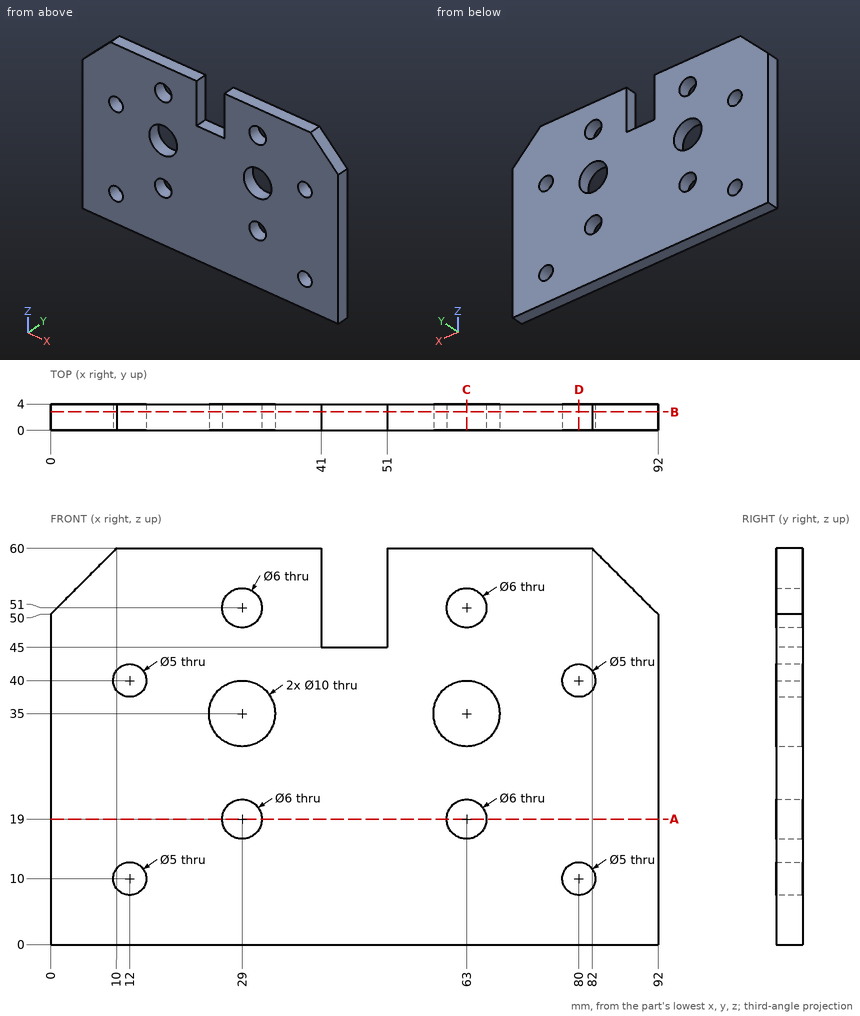
Check sheet for the drawn part. Datum: minimum x, y, z corner. Units: mm. Round coordinates to 2 decimals unless told otherwise and drop trailing zeros. Loops run counter-clockwise (first coordinate to the right, second up) from the corner with the lowest first, then second, coordinate; pieces in that order, holes last.
Item 1: Gauge pin test, flat ends, axial feed: pin 1 (7 mm diameter, centred on x = 63, z = 19, fed in from -Y); pin 2 (5.5 mm diameter, centred on x = 63, z = 51, fed in from -Y) (1 decimal); pin 3 (2 mm diameter, centred on y = 2, z = 53, fed in from -X); pin 4 (1.2 mm diameter, centred on y = 2.5, z = 54, fed in from +X). Record the tip position at first contact, or that the pin passes through.
Item 2: Cross-section at C-C on x = 63. Record the boundary of the cut face in (y, z), then the cut area to 3 significant figures.
Item 3: Cross-section at D-D on x = 80. Record the boundary of the cut face in (y, z).
Item 4: Thickness scan on line 1 (X direction, y = 1.2, z = 35); line 2 (X direction, y = 1.2, z = 19); line 3 (X direction, y = 0.6, z = 47). Record the ranges inside material, lowest first.
Item 5: Cross-section at A-A on z = 19. Record the boundary of the cut face in (x, y).
Item 6: Cross-section at B-B on y = 2.8. Count the separate pieces of the cut face and the enclosed holes in it, then the cut area to 3 significant figures.
Answer sheet:
1. pin 1: stops at y = 0
1. pin 2: passes through
1. pin 3: stops at x = 2
1. pin 4: stops at x = 88.6
2. outline: (0, 0) - (4, 0) - (4, 16) - (0, 16) - close; (0, 22) - (4, 22) - (4, 30) - (0, 30) - close; (0, 40) - (4, 40) - (4, 48) - (0, 48) - close; (0, 54) - (4, 54) - (4, 60) - (0, 60) - close
2. area: 152 mm2
3. outline: (0, 0) - (4, 0) - (4, 7.5) - (0, 7.5) - close; (0, 12.5) - (4, 12.5) - (4, 37.5) - (0, 37.5) - close; (0, 42.5) - (4, 42.5) - (4, 60) - (0, 60) - close
4. line 1: x = 0 to 24, 34 to 58, 68 to 92
4. line 2: x = 0 to 26, 32 to 60, 66 to 92
4. line 3: x = 0 to 41, 51 to 92
5. outline: (0, 0) - (26, 0) - (26, 4) - (0, 4) - close; (32, 0) - (60, 0) - (60, 4) - (32, 4) - close; (66, 0) - (92, 0) - (92, 4) - (66, 4) - close
6. separate pieces: 1
6. enclosed holes: 10
6. area: 4,920 mm2
